from build123d import *

# Parameters (mm, degrees)
CROQUIS1_W              = 26
CROQUIS1_H              = 6
CROQUIS1_R              = 1.75
SALIENTE_EXTRUIR1_DEPTH = 4
REDONDEO2_R             = 3


with BuildPart() as part:
    # Croquis1 → Saliente-Extruir1 (new body)
    with BuildSketch(Plane.XY):
        with Locations((-8.309993141, 2.824852585)):
            Rectangle(CROQUIS1_W, CROQUIS1_H)
        with Locations((1.690006859, 2.824852585)):
            Circle(CROQUIS1_R, mode=Mode.SUBTRACT)
        with Locations((-18.309993141, 2.824852585)):
            Circle(CROQUIS1_R, mode=Mode.SUBTRACT)
    extrude(amount=SALIENTE_EXTRUIR1_DEPTH)

    # Redondeo2
    redondeo2_edges = [part.edges().sort_by_distance(p)[0] for p in [
        (4.690006859, 5.824852585, 2),
        (4.690006859, -0.175147415, 2),
        (-21.309993141, 5.824852585, 2),
        (-21.309993141, -0.175147415, 2),
    ]]
    fillet(redondeo2_edges, radius=REDONDEO2_R - 0.0001)  # a hair under: the kernel refuses the full size


solid = part.part
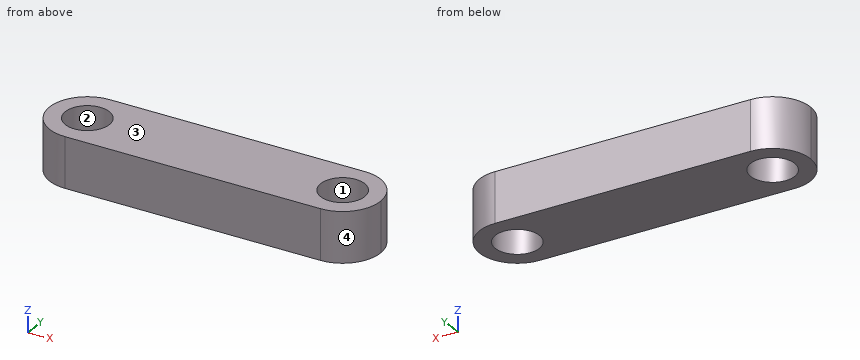
Work out the finished part from the listing and answer in its coordinate system (mm). Face numbers are marked on the shaded views. Give positions to 0.01 mm unless a question says otherwise; leave off trailing zeros. Loops run counter-clockwise (first coordinate to the right, second up) from the corner with the lowest first, then second, coordinate; pieces in that order, holes last. Notation, with made-up numbers: (37.5, 60) -> (69.5, 60) arc R12 ccw to (69.5, 70) -> close; hole circle Ø8 at (-26.5, 73.5). An arc over 180 degrees is marked (long way). Use a Markdown table: item, result. Add a question column.
1. Section C-C on z = 2.4 is taken. State how many separate pieces and enclosed holes the cut face has, and give its area (3 significant figures).
2. Section A-A on x = -19 is taken. Determine the outline of the cut face in (y, z), and give its area (3 significant figures).
3. Determine the mould class of the marked faces 1, 2, 3 and 4 for opening direction X: released by +X, released by -X, zero draft, split by the parting line, or undercut.
4. Find the intervals of material crossed by probe 1 along X at (y, z) = (2.75, 2.9); probe 2 along X at (y, z) = (3.25, 0.9); probe 3 along Y at (x, z) = (-18.25, 2.7), in increasing order.
5. A flat-ended cylindrical pin translates along its axis: pin 1 Ø3 at (x, y) = (1.69, 2.82) entering from -Z. Find the tip coordinate at first contact, or state that the pin passes through.
6. Section B-B on y = 1.5 is taken. Determine the outline of the cut face in (x, z).
7. Section D-D on y = 2.5 is taken. Determine the outline of the cut face in (x, z), and give its area (3 significant figures).
Results below:
| question | item | result |
|---|---|---|
| 1 | separate pieces | 1 |
| 1 | enclosed holes | 2 |
| 1 | area | 129 mm^2 |
| 2 | outline | (-0.09, 0) -> (1.22, 0) -> (1.22, 4) -> (-0.09, 4) -> close; (4.43, 0) -> (5.74, 0) -> (5.74, 4) -> (4.43, 4) -> close |
| 2 | area | 10.5 mm^2 |
| 3 | face 1 | undercut |
| 3 | face 2 | undercut |
| 3 | face 3 | zero draft |
| 3 | face 4 | released by +X |
| 4 | probe 1 | x = -21.31 to -20.06, -16.56 to -0.06, 3.44 to 4.69 |
| 4 | probe 2 | x = -21.28 to -20.01, -16.61 to -0.01, 3.39 to 4.66 |
| 4 | probe 3 | y = -0.18 to 1.08, 4.57 to 5.82 |
| 5 | pin 1 | passes through |
| 6 | outline | (-21, 0) -> (-19.45, 0) -> (-19.45, 4) -> (-21, 4) -> close; (-17.17, 0) -> (0.55, 0) -> (0.55, 4) -> (-17.17, 4) -> close; (2.83, 0) -> (4.38, 0) -> (4.38, 4) -> (2.83, 4) -> close |
| 7 | outline | (-21.29, 0) -> (-20.03, 0) -> (-20.03, 4) -> (-21.29, 4) -> close; (-16.59, 0) -> (-0.03, 0) -> (-0.03, 4) -> (-16.59, 4) -> close; (3.41, 0) -> (4.67, 0) -> (4.67, 4) -> (3.41, 4) -> close |
| 7 | area | 76.3 mm^2 |
